```python
from build123d import *

# Parameters (mm, degrees)
CROQUIS1_R              = 1.35
CROQUIS1_R_2            = 4
SALIENTE_EXTRUIR1_DEPTH = 4
CROQUIS2_R              = 3
CROQUIS2_R_2            = 1
CORTAR_EXTRUIR1_DEPTH   = 4
REDONDEO1_R             = 1.6
CROQUIS3_R              = 1
CORTAR_EXTRUIR2_DEPTH   = 4


with BuildPart() as part:
    # Croquis1 → Saliente-Extruir1 (new body)
    with BuildSketch(Plane.XY):
        with BuildLine():
            Line((-15, -10.656453444), (-15, -37.656453444))
            Line((-15, -37.656453444), (15, -37.656453444))
            Line((15, -37.656453444), (15, -10.656453444))
            ThreePointArc((15, -10.656453444), (0, 18.4), (-15, -10.656453444))
        make_face()
        with Locations((-7.071067812, -7.071067812)):
            Circle(CROQUIS1_R, mode=Mode.SUBTRACT)
        with Locations((-7.071067812, 7.071067812)):
            Circle(CROQUIS1_R, mode=Mode.SUBTRACT)
        with Locations((7.071067812, 7.071067812)):
            Circle(CROQUIS1_R, mode=Mode.SUBTRACT)
        with Locations((7.071067812, -7.071067812)):
            Circle(CROQUIS1_R, mode=Mode.SUBTRACT)
        Circle(CROQUIS1_R_2, mode=Mode.SUBTRACT)
        with Locations((-10, -34.656453444)):
            Circle(CROQUIS1_R, mode=Mode.SUBTRACT)
        with Locations(Location((10, -34.656453444, 0), (0, 0, 180))):
            Circle(CROQUIS1_R, mode=Mode.SUBTRACT)
    extrude(amount=SALIENTE_EXTRUIR1_DEPTH)

    # Croquis2 → Cortar-Extruir1 (cut)
    with BuildSketch(Plane.XY.offset(4)):
        with Locations((7, -27.656453444)):
            Circle(CROQUIS2_R)
        with Locations((5.211145618, -21.234162208)):
            Circle(CROQUIS2_R_2)
        with Locations(Location((8.788854382, -21.234162208, 0), (0, 0, 180))):
            Circle(CROQUIS2_R_2)
    extrude(amount=-CORTAR_EXTRUIR1_DEPTH, mode=Mode.SUBTRACT)

    # Redondeo1
    redondeo1_edges = [part.edges().sort_by_distance(p)[0] for p in [
        (15, -10.656453444, 2),
        (15, -37.656453444, 2),
        (-15, -37.656453444, 2),
        (-15, -10.656453444, 2),
    ]]
    fillet(redondeo1_edges, radius=REDONDEO1_R)

    # Croquis3 → Cortar-Extruir2 (cut)
    with BuildSketch(Plane.XY.offset(4)):
        with Locations((0, -23.156453444)):
            Circle(CROQUIS3_R)
    extrude(amount=-CORTAR_EXTRUIR2_DEPTH, mode=Mode.SUBTRACT)


solid = part.part
```
Input: part model. Units: mm. Frame: model coordinates. A direction names the side the tool comes from. Give positions to 0.01 mm unless a question says otherwise; leave off trailing zeros. Order: outer loops, then holes, each group sorted by start corner. A loop starts at its lowest first (then second) coordinate and runs counter-clockwise, first axis right, second up.
1. Section A-A on y = 0. Return the cut outline in (x, z), and give its area (3 significant figures).
Derived:
outline: (-18.4, 0) - (-4, 0) - (-4, 4) - (-18.4, 4) - close; (4, 0) - (18.4, 0) - (18.4, 4) - (4, 4) - close
area: 115 mm2
2. Material intervals for L1, parallel to Y at x = 0, z = 1.4; L2, parallel to Y at x = 5, z = 1.75; L3, parallel to X at y = -23, z = 2.05, sorted ascending.
Derived:
L1: y = -37.66 to -24.16, -22.16 to -4, 4 to 18.4
L2: y = -37.66 to -29.89, -25.42 to -22.21, -20.26 to 17.71
L3: x = -15 to -0.99, 0.99 to 15
3. Section D-D on x = -10. Return the cut outline in (y, z).
Derived:
outline: (-37.66, 0) - (-36.01, 0) - (-36.01, 4) - (-37.66, 4) - close; (-33.31, 0) - (15.45, 0) - (15.45, 4) - (-33.31, 4) - close
4. Section B-B on x = 0. Return the cut outline in (y, z), and give its area (3 significant figures).
Derived:
outline: (-37.66, 0) - (-24.16, 0) - (-24.16, 4) - (-37.66, 4) - close; (-22.16, 0) - (-4, 0) - (-4, 4) - (-22.16, 4) - close; (4, 0) - (18.4, 0) - (18.4, 4) - (4, 4) - close
area: 184 mm2
5. Reachability of faces 1 (the flat face through (15, -24, 2)), 2 (the cylindrical face through (10.176, -35.995, 1.972)) from +Z, -Z, +X, -X, +Y, -Y: full face, straight path, thin tool, end or side. Return the list, or none.
Derived:
face 1: +Z, -Z, +X, -Y
face 2: +Z, -Z
6. Section C-C on z = 1.8. Give the number of separate pieces and of enclosed holes in the cut face, and give its area (3 significant figures).
Derived:
separate pieces: 1
enclosed holes: 11
area: 1,590 mm2
7. Mould query, pull axis Y, two halves, no side actions, for faces 3 (the cylindrical face through (-0.867, -3.905, 1.972)), 4 (the flat face through (-15, -23, 2)), 5 (the cylindrical face through (0.56, 18.39, 1.97)). Classes: released by +Y, released by -Y, zero draft, split by the parting line, or undercut.
Derived:
face 3: undercut
face 4: zero draft
face 5: split by the parting line
8. Pin query (flat end, axial travel): pin 1 (1.2 mm diameter, centred on y = -17.5, z = 2.5, fed in from -X); pin 2 (1.5 mm diameter, centred on y = 7, z = 1.5, fed in from -X); pin 3 (1.2 mm diameter, centred on y = -22, z = 2.5, fed in from +X). Return the tip coordinate at first contact, or that it passes through.
Derived:
pin 1: stops at x = -15
pin 2: stops at x = -17.31
pin 3: stops at x = 15
